from build123d import *

# Parameters (mm, degrees)
SKETCH1_W           = 50.8
SKETCH1_H           = 50.8
BOSS_EXTRUDE1_DEPTH = 6.35
CUT_EXTRUDE6_DEPTH  = 73.122135992


with BuildPart() as part:
    # Sketch1 → Boss-Extrude1 (new body)
    with BuildSketch(Plane(origin=(0, 0, 0), x_dir=(1, 0, 0), z_dir=(0, 1, 0))):
        with Locations((25.4, 25.4)):
            Rectangle(SKETCH1_W, SKETCH1_H)
    extrude(amount=BOSS_EXTRUDE1_DEPTH)

    # Sketch2 → Cut-Extrude6 (cut, through all)
    with BuildSketch(Plane(origin=(0, 6.35, 0), x_dir=(1, 0, 0), z_dir=(0, 1, 0))):
        Polygon((21.59, 47.625), (23.8125, 47.625), (23.8125, 50.8), (26.9875, 50.8), (26.9875, 47.625), (29.21, 47.625), (29.21, 44.45), (26.9875, 44.45), (26.9875, 41.275), (23.8125, 41.275), (23.8125, 44.45), (21.59, 44.45), align=None)
        Polygon((26.9875, 6.35), (29.21, 6.35), (29.21, 3.175), (26.9875, 3.175), (26.9875, 0), (23.8125, 0), (23.8125, 3.175), (21.59, 3.175), (21.59, 6.35), (23.8125, 6.35), (23.8125, 9.525), (26.9875, 9.525), align=None)
        Polygon((3.175, 26.9875), (3.175, 29.21), (6.35, 29.21), (6.35, 26.9875), (9.525, 26.9875), (9.525, 23.8125), (6.35, 23.8125), (6.35, 21.59), (3.175, 21.59), (3.175, 23.8125), (0, 23.8125), (0, 26.9875), align=None)
        Polygon((47.625, 23.8125), (50.8, 23.8125), (50.8, 26.9875), (47.625, 26.9875), (47.625, 29.21), (44.45, 29.21), (44.45, 26.9875), (41.275, 26.9875), (41.275, 23.8125), (44.45, 23.8125), (44.45, 21.59), (47.625, 21.59), align=None)
    extrude(amount=-CUT_EXTRUDE6_DEPTH, mode=Mode.SUBTRACT)


solid = part.part
Design review of the part built by this model. Coordinates are the model's own, in mm. A direction names the side the tool comes from. Give positions to 0.01 mm unless a question says otherwise; leave off trailing zeros. Order: outer loops, then holes, each group sorted by start corner. A loop starts at its lowest first (then second) coordinate and runs counter-clockwise, first axis right, second up. Notation, with made-up numbers: (74, 61.5) - (101, 61.5) arc R10 cw to (101, 73.5) - close; hole circle Ø4 at (57.25, 57.5). An arc over 180 degrees is marked (long way). Write item = value, one per line. Start each with the question number.
Q1. Mouldability with a two-part tool opening along X and no side actions: class faces 1 (the face through (39, 3, -50.8)), 2 (the face through (26.988, 3, -43)) as released by +X, released by -X, zero draft, split by the parting line, or undercut.
Q2. We need section C-C on x = 26. State the section outline as (y, z) points (3 decimals).
Q3. To check wall thickness, follow L1, parallel to X at y = 4.5, z = -28.5 (3 decimals); L2, parallel to Z at x = 7.5, y = 0.5; L3, parallel to Z at x = 3.5, y = 2.5. State the ranges of each line that lie inside material, in increasing order. Write a range as from..to.
Q4. Tool access review of faces 3 (the face through (5, 3, -21.59)), 4 (the face through (26.988, 3, -49)), 5 (the face through (26.988, 3, -8)): name each direction out of +Z, -Z, +X, -X, +Y, -Y from which nothing blocks a thin tool from reaching the whole face with its end or side.
Q5. We need section A-A on x = 5. State the section outline as (y, z) points.
Q6. Clearance check with flat-ended pins moving along their axes: pin 1 Ø1 at (x, y) = (8.5, 5.5) entering from +Z; pin 2 Ø1 at (x, y) = (24.5, 1.5) entering from -Z (3 decimals); pin 3 Ø1 at (y, z) = (4.5, -25.5) entering from -X (3 decimals). State where each tip first meets the part, or that it passes through.
Q7. We need section B-B on z = -4.5. State the section outline as (x, y) points.
Working result:
q1.face_1 = zero draft
q1.face_2 = undercut
q2.outline = (0, -41.275) - (6.35, -41.275) - (6.35, -9.525) - (0, -9.525) - close
q3.L1 = 0..3.175, 6.35..44.45, 47.625..50.8
q3.L2 = -50.8..-26.99, -23.81..0
q3.L3 = -50.8..-29.21, -21.59..0
q4.face_3 = +Y, -Y
q4.face_4 = -Z, +Y, -Y
q4.face_5 = +Z, +Y, -Y
q5.outline = (0, -50.8) - (6.35, -50.8) - (6.35, -29.21) - (0, -29.21) - close; (0, -21.59) - (6.35, -21.59) - (6.35, 0) - (0, 0) - close
q6.pin_1 = 0
q6.pin_2 = -41.275
q6.pin_3 = 9.525
q7.outline = (0, 0) - (21.59, 0) - (21.59, 6.35) - (0, 6.35) - close; (29.21, 0) - (50.8, 0) - (50.8, 6.35) - (29.21, 6.35) - close
